from build123d import *

# Parameters (mm, degrees)
SKETCH1_W           = 15
SKETCH1_H           = 15
BOSS_EXTRUDE1_DEPTH = 4.5
SKETCH2_W           = 12
SKETCH2_H           = 12
CUT_EXTRUDE1_DEPTH  = 3.5
SKETCH3_R           = 1.25
BOSS_EXTRUDE2_DEPTH = 2
FILLET1_R           = 1
SKETCH4_R           = 0.5
BOSS_EXTRUDE3_DEPTH = 2


with BuildPart() as part:
    # Sketch1 → Boss-Extrude1 (new body)
    with BuildSketch(Plane(origin=(0, 0, 0), x_dir=(1, 0, 0), z_dir=(0, 1, 0))):
        Rectangle(SKETCH1_W, SKETCH1_H)
    extrude(amount=BOSS_EXTRUDE1_DEPTH)

    # Sketch2 → Cut-Extrude1 (cut)
    with BuildSketch(Plane(origin=(0, 4.5, 0), x_dir=(1, 0, 0), z_dir=(0, 1, 0))):
        Rectangle(SKETCH2_W, SKETCH2_H)
    extrude(amount=-CUT_EXTRUDE1_DEPTH, mode=Mode.SUBTRACT)

    # Sketch3 → Boss-Extrude2 (add)
    with BuildSketch(Plane(origin=(0, 1, 0), x_dir=(1, 0, 0), z_dir=(0, 1, 0))):
        Circle(SKETCH3_R)
    extrude(amount=BOSS_EXTRUDE2_DEPTH)

    # Fillet1
    fillet1_edges = [part.edges().sort_by_distance(p)[0] for p in [
        (-1.25, 3, 0),
    ]]
    fillet(fillet1_edges, radius=FILLET1_R)

    # Sketch4 → Boss-Extrude3 (add)
    with BuildSketch(Plane(origin=(0, 4.5, 0), x_dir=(1, 0, 0), z_dir=(0, 1, 0))):
        with Locations((-6.7, 6.7)):
            Circle(SKETCH4_R)
        with Locations((6.7, 6.7)):
            Circle(SKETCH4_R)
        with Locations((6.7, -6.7)):
            Circle(SKETCH4_R)
        with Locations((-6.7, -6.7)):
            Circle(SKETCH4_R)
    extrude(amount=BOSS_EXTRUDE3_DEPTH)


solid = part.part
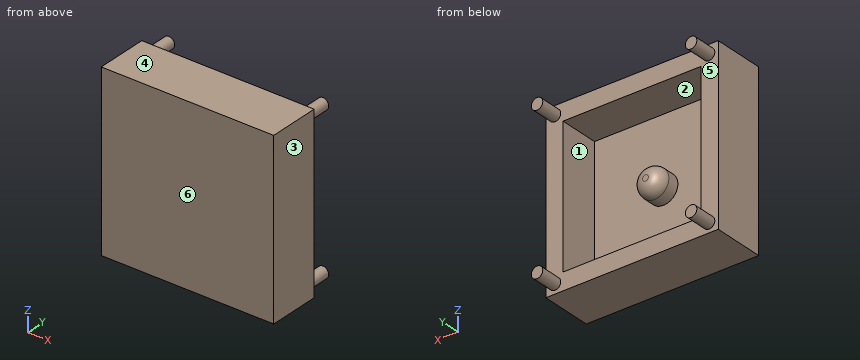
Check sheet for the modelled part. Datum: model origin and axes. Units: mm. Face numbers are marked on the shaded views. A direction names the side the tool comes from. Give positions to 0.01 mm unless a question says otherwise; leave off trailing zeros. Loops run counter-clockwise (first coordinate to the right, second up) from the corner with the lowest first, then second, coordinate; pieces in that order, holes last. Notation, with made-up numbers: M 30.25,54.25 L 53.25,54.25 A10 ccw 53.25,60.25 Z; hole C -2.75,36.5 d4. An arc over 180 degrees is marked long. Return JSON: item names as keys, results as strings. Group by question number.
1. Thickness scan on L1, parallel to X at y = 1.5, z = -5.75; L2, parallel to Y at x = -3.25, z = 1.75; L3, parallel to Y at x = -5.25, z = 6.5. Record the ranges inside material, lowest first.
2. Go/stop test with flat-tipped pins: pin 1 (3.5 mm diameter, centred on x = -3, z = -1.5, fed in from +Y); pin 2 (2 mm diameter, centred on x = -3.5, z = -5.5, fed in from +Y); pin 3 (8 mm diameter, centred on x = -4, z = -6, fed in from -Y). Record where each tip stops, or that it passes through.
3. Cross-section at C-C on x = 6.7. Record the boundary of the cut face in (y, z), plus the area to 3 significant figures.
4. Cross-section at B-B on y = 4. Record the boundary of the cut face in (x, z).
5. Cross-section at A-A on y = 1.75. Record the boundary of the cut face in (x, z), plus the area to 3 significant figures.
6. Tool access check on the marked faces 5 and 6. Record the directions out of +Z, -Z, +X, -X, +Y, -Y that give a thin tool (end or side, any length) a straight path to the whole face; none if there is none.
7. Cross-section at D-D on z = -6.7. Record the boundary of the cut face in (x, y).
8. Mould release check, pull along X, two halves, no side actions. Record for the marked faces 1, 2, 3 and 4: released by +X, released by -X, zero draft, split by the parting line, or undercut.
Return value:
{
 "1": {"L1": "-7.5 to -6, 6 to 7.5", "L2": "0 to 1", "L3": "0 to 4.5"},
 "2": {"pin 1": "y = 1", "pin 2": "y = 4.5", "pin 3": "y = 0"},
 "3": {"outline": "M 0,-7.5 L 4.5,-7.5 L 4.5,-7.2 L 6.5,-7.2 L 6.5,-6.2 L 4.5,-6.2 L 4.5,6.2 L 6.5,6.2 L 6.5,7.2 L 4.5,7.2 L 4.5,7.5 L 0,7.5 Z", "area": "71.5 mm^2"},
 "4": {"outline": "M -7.5,-7.5 L 7.5,-7.5 L 7.5,7.5 L -7.5,7.5 Z; hole M -6,-6 L 6,-6 L 6,6 L -6,6 Z"},
 "5": {"outline": "M -7.5,-7.5 L 7.5,-7.5 L 7.5,7.5 L -7.5,7.5 Z; C 0,0 d2.5; hole M -6,-6 L 6,-6 L 6,6 L -6,6 Z", "area": "85.9 mm^2"},
 "6": {"face 5": "+Y", "face 6": "+Z, -Z, +X, -X, -Y"},
 "7": {"outline": "M -7.5,0 L 7.5,0 L 7.5,4.5 L 7.2,4.5 L 7.2,6.5 L 6.2,6.5 L 6.2,4.5 L -6.2,4.5 L -6.2,6.5 L -7.2,6.5 L -7.2,4.5 L -7.5,4.5 Z"},
 "8": {"face 1": "undercut", "face 2": "undercut", "face 3": "released by +X", "face 4": "zero draft"}
}
